For this review, use the dimensioned drawing (mm, ordinates from the lowest corner) and the shaded views. A direction names the side the tool comes from. Give positions to 0.01 mm unless a question says otherwise; leave off trailing zeros. Loops run counter-clockwise (first coordinate to the right, second up) from the corner with the lowest first, then second, coordinate; pieces in that order, holes last. Notation, with made-up numbers: (8.25, 72) - (29.25, 72) arc R22 cw to (29.25, 80) - close; hole circle Ø11 at (-38, 1). An arc over 180 degrees is marked (long way). Put each result on its own line as item: value.
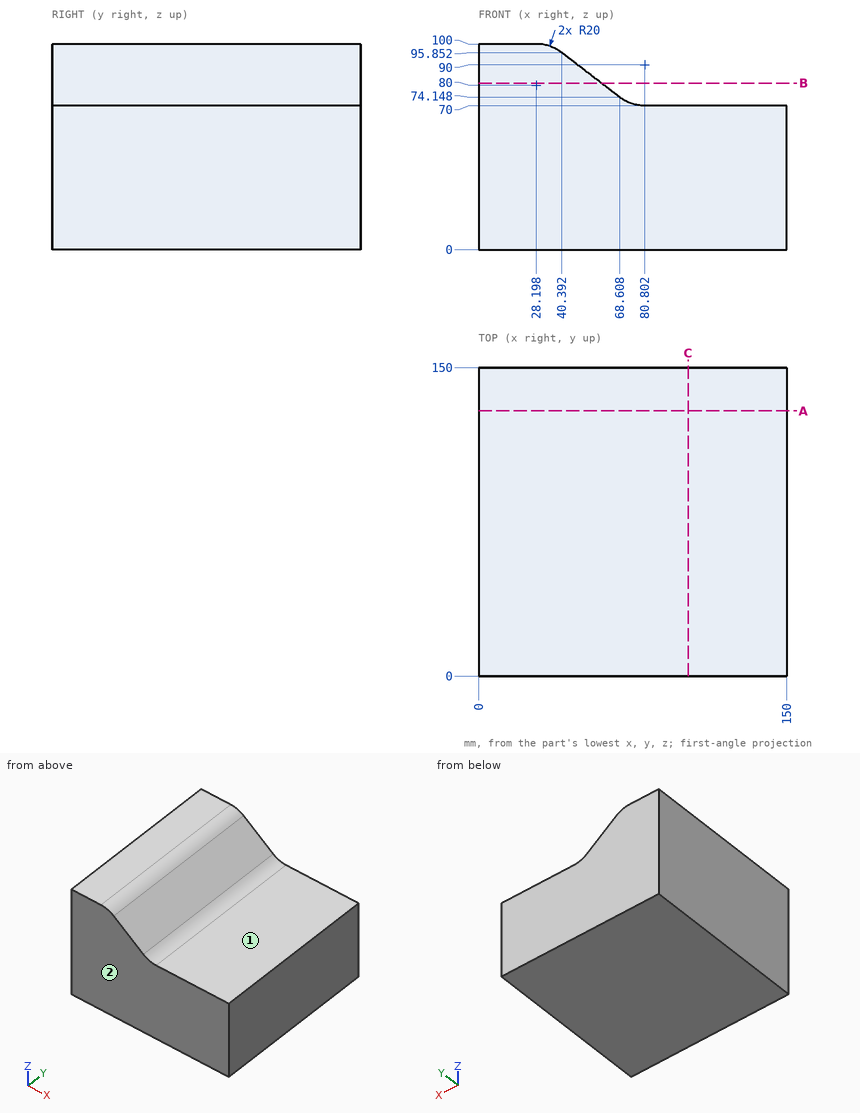
1) Take a section at A-A on y = 129. State the section outline as (x, z) points.
Geometry check:
outline: (0, 0) - (150, 0) - (150, 70) - (80.8, 70) arc R20 cw to (68.61, 74.15) - (40.39, 95.85) arc R20 ccw to (28.2, 100) - (0, 100) - close
2) Wall thickness on line 1 (Z direction, x = 129, y = 88); line 2 (X direction, y = 76, z = 78); line 3 (X direction, y = 91, z = 91): over which ranges is each line inside the solid? List them lowest first.
Geometry check:
line 1: z = 0 to 70
line 2: x = 0 to 63.6
line 3: x = 0 to 46.7
3) Insertion check: pin 1 Ø21 at (x, y) = (110.5, 111) entering from +Z; pin 2 Ø2 at (x, y) = (80, 96.5) entering from +Z. Each pin has a flat end and moves straight along its axis. Give the tip position at first contact, or say it passes through.
Geometry check:
pin 1: stops at z = 70
pin 2: stops at z = 70.08
4) For the marked faces 1 and 2, list the 3-axis set-ups (+Z, -Z, +X, -X, +Y, -Y) from which the entire face can be reached by the end or side of a thin tool; tool diameter is ignored.
Geometry check:
face 1: +Z, +X, +Y, -Y
face 2: +Z, -Z, +X, -X, -Y
5) Take a section at C-C on x = 102. State the section outline as (y, z) points.
Geometry check:
outline: (0, 0) - (150, 0) - (150, 70) - (0, 70) - close
6) Take a section at B-B on z = 81. State the section outline as (x, y) points, and give its area (4 significant figures).
Geometry check:
outline: (0, 0) - (59.7, 0) - (59.7, 150) - (0, 150) - close
area: 8,955 mm²
